Check sheet for the modelled part. Datum: model origin and axes. Units: mm. A direction names the side the tool comes from. Round coordinates to 2 decimals unless told otherwise and drop trailing zeros. Write each loop counter-clockwise with the first axis right and the second up, starting at its lowest first coordinate (ties: lowest second). Pieces come first, ordered by that corner, then holes. Notation, with made-up numbers: M -14.5,30.5 L 27.5,30.5 A6 ccw 27.5,39.5 Z; hole C 84.25,78.25 d11. An arc over 180 degrees is marked long. One line per item, written item: value.
from build123d import *

# Parameters (mm, degrees)
ESQUISSE1_W              = 80
ESQUISSE1_H              = 80
BOSS_EXTRU_1_DEPTH       = 20
ESQUISSE2_W              = 76
ESQUISSE2_H              = 76
BOSS_EXTRU_2_DEPTH       = 5
ESQUISSE3_W              = 72
ESQUISSE3_H              = 72
ENL_V_MAT_EXTRU_2_DEPTH  = 23
ESQUISSE4_W              = 15
ESQUISSE4_H              = 17.5
ESQUISSE4_W_2            = 17.5
ESQUISSE4_H_2            = 15
ENL_V_MAT_EXTRU_9_DEPTH  = 10
ESQUISSE7_R              = 2.5
ENL_V_MAT_EXTRU_4_DEPTH  = 10
ESQUISSE5_R              = 5
BOSS_EXTRU_6_DEPTH       = 10
ESQUISSE9_R              = 2
ENL_V_MAT_EXTRU_6_DEPTH  = 8
ESQUISSE10_W             = 2
ESQUISSE10_H             = 10
ENL_V_MAT_EXTRU_7_DEPTH  = 5
ESQUISSE11_OUTSIDE_W     = 105.174
ESQUISSE11_OUTSIDE_H     = 105.174
ESQUISSE11_OUTSIDE_W_2   = 75.6
ESQUISSE11_OUTSIDE_H_2   = 75.6
ENL_V_MAT_EXTRU_10_DEPTH = 3
BOSS_EXTRU_7_REACH       = 131.891
BOSS_EXTRU_7_START       = -15
ENL_V_MAT_EXTRU_11_DEPTH = 3


with BuildPart() as part:
    # Esquisse1 → Boss.-Extru.1 (new body)
    with BuildSketch(Plane(origin=(0, 0, 0), x_dir=(1, 0, 0), z_dir=(0, 1, 0))):
        with Locations((40, -40)):
            Rectangle(ESQUISSE1_W, ESQUISSE1_H)
    extrude(amount=BOSS_EXTRU_1_DEPTH)

    # Esquisse2 → Boss.-Extru.2 (add)
    with BuildSketch(Plane(origin=(0, 20, 0), x_dir=(1, 0, 0), z_dir=(0, 1, 0))):
        with Locations((40, -40)):
            Rectangle(ESQUISSE2_W, ESQUISSE2_H)
    extrude(amount=BOSS_EXTRU_2_DEPTH)

    # Esquisse3 → Enlèv. mat.-Extru.2 (cut)
    with BuildSketch(Plane(origin=(0, 25, 0), x_dir=(1, 0, 0), z_dir=(0, 1, 0))):
        with Locations((40, -40)):
            Rectangle(ESQUISSE3_W, ESQUISSE3_H)
    extrude(amount=-ENL_V_MAT_EXTRU_2_DEPTH, mode=Mode.SUBTRACT)

    # Esquisse4 → Enlèv. mat.-Extru.9 (cut)
    with BuildSketch(Plane.XZ):
        with Locations((40, 23.75)):
            Rectangle(ESQUISSE4_W, ESQUISSE4_H)
        with Locations((23.75, 40)):
            Rectangle(ESQUISSE4_W_2, ESQUISSE4_H_2)
        with Locations((40, 40)):
            Rectangle(ESQUISSE4_W, ESQUISSE4_H_2)
        with Locations((56.25, 40)):
            Rectangle(ESQUISSE4_W_2, ESQUISSE4_H_2)
        with Locations((40, 56.25)):
            Rectangle(ESQUISSE4_W, ESQUISSE4_H)
    extrude(amount=-ENL_V_MAT_EXTRU_9_DEPTH, mode=Mode.SUBTRACT)

    # Esquisse7 → Enlèv. mat.-Extru.4 (cut)
    with BuildSketch(Plane(origin=(0, 0, 0), x_dir=(-1, 0, 0), z_dir=(0, -1, 0))):
        with Locations(Location((-15, -15, 0), (0, 0, 90))):
            Circle(ESQUISSE7_R)
        with Locations(Location((-15, -65, 0), (0, 0, 90))):
            Circle(ESQUISSE7_R)
        with Locations(Location((-65, -15, 0), (0, 0, 90))):
            Circle(ESQUISSE7_R)
        with Locations(Location((-65, -65, 0), (0, 0, 90))):
            Circle(ESQUISSE7_R)
    extrude(amount=-ENL_V_MAT_EXTRU_4_DEPTH, mode=Mode.SUBTRACT)

    # Esquisse5 → Boss.-Extru.6 (add)
    with BuildSketch(Plane(origin=(0, 0, 0), x_dir=(-1, 0, 0), z_dir=(0, -1, 0))):
        with Locations(Location((-55, -25, 0), (0, 0, 90))):
            Circle(ESQUISSE5_R)
        with Locations(Location((-55, -55, 0), (0, 0, 90))):
            Circle(ESQUISSE5_R)
        with Locations(Location((-25, -55, 0), (0, 0, 90))):
            Circle(ESQUISSE5_R)
        with Locations(Location((-25, -25, 0), (0, 0, 90))):
            Circle(ESQUISSE5_R)
    extrude(amount=-BOSS_EXTRU_6_DEPTH)

    # Esquisse9 → Enlèv. mat.-Extru.6 (cut)
    with BuildSketch(Plane(origin=(0, 0, 0), x_dir=(-1, 0, 0), z_dir=(0, -1, 0))):
        with Locations(Location((-55, -25, 0), (0, 0, 90))):
            Circle(ESQUISSE9_R)
        with Locations(Location((-55, -55, 0), (0, 0, 90))):
            Circle(ESQUISSE9_R)
        with Locations(Location((-25, -25, 0), (0, 0, 90))):
            Circle(ESQUISSE9_R)
        with Locations(Location((-25, -55, 0), (0, 0, 90))):
            Circle(ESQUISSE9_R)
    extrude(amount=-ENL_V_MAT_EXTRU_6_DEPTH, mode=Mode.SUBTRACT)

    # Esquisse10 → Enlèv. mat.-Extru.7 (cut)
    with BuildSketch(Plane(origin=(0, 25, 0), x_dir=(1, 0, 0), z_dir=(0, 1, 0))):
        with Locations((3, -21)):
            Rectangle(ESQUISSE10_W, ESQUISSE10_H)
    extrude(amount=-ENL_V_MAT_EXTRU_7_DEPTH, mode=Mode.SUBTRACT)

    # Esquisse11 outside → Enlèv. mat.-Extru.10 (cut)
    with BuildSketch(Plane(origin=(0, 0, 0), x_dir=(-1, 0, 0), z_dir=(0, -1, 0))):
        with Locations((-40, -40)):
            Rectangle(ESQUISSE11_OUTSIDE_W, ESQUISSE11_OUTSIDE_H)
        with Locations((-40, -40)):
            Rectangle(ESQUISSE11_OUTSIDE_W_2, ESQUISSE11_OUTSIDE_H_2, mode=Mode.SUBTRACT)
    extrude(amount=-ENL_V_MAT_EXTRU_10_DEPTH, mode=Mode.SUBTRACT)

    # Esquisse14 → Boss.-Extru.7 (add, up to next)
    with BuildSketch(Plane(origin=(0, 20, 0), x_dir=(1, 0, 0), z_dir=(0, 1, 0)).offset(BOSS_EXTRU_7_START), mode=Mode.PRIVATE) as boss_extru_7_sk1:
        Polygon((76, -76), (76, -65.703145172), (66.703318607, -76), align=None)
    boss_extru_7_tool1 = extrude(boss_extru_7_sk1.sketch, amount=-BOSS_EXTRU_7_REACH, mode=Mode.PRIVATE) - part.part
    add(boss_extru_7_tool1.solids().sort_by_distance((72.901106, 5, 72.567715))[0])

    # Esquisse13 → Enlèv. mat.-Extru.11 (cut)
    with BuildSketch(Plane(origin=(0, 0, 0), x_dir=(-1, 0, 0), z_dir=(0, -1, 0))):
        Polygon((-63.5, -80), (-80, -63.5), (-80, -80), align=None)
    extrude(amount=-ENL_V_MAT_EXTRU_11_DEPTH, mode=Mode.SUBTRACT)


solid = part.part
Q1. Sectioned sample at B-B on y = 9. Enter the section's corners in (x, z), and give its area (3 significant figures).
Completed:
outline: M 0,0 L 80,0 L 80,80 L 0,80 Z; C 25,25 d10; C 25,55 d10; C 55,25 d10; C 55,55 d10; hole M 4,4 L 76,4 L 76,76 L 4,76 Z
area: 1,530 mm^2
Q2. Scan lines: line 1 (X direction, y = 3.25, z = 55); line 2 (X direction, y = 7.75, z = 35.5). Record each from-to range of solid material in increasing order. Write a range as [from, to].
Completed:
line 1: [0, 4], [20, 23], [27, 30], [50, 53], [57, 60], [76, 80]
line 2: [0, 4], [76, 80]
Q3. Depth check by flat-ended pin: P1, Ø11, axis at x = 55, z = 53, coming from the +Y side; P2, Ø2.5, axis at y = 2, z = 51.5, coming from the -X side; P3, Ø1.2, axis at x = 25.5, z = 55, coming from the -Y side; P4, Ø1.5, axis at x = 22.5, y = 23, coming from the +Z side. Enter the tip coordinate at first touch or a pass-through.
Completed:
P1: y = 10
P2: x = 0
P3: y = 8
P4: z = 78
Q4. Access from +Z, -Z, +X, -X, +Y, -Y to the whole of each face (thin tool, end or side, straight path). Record for faces 1 (the flat face through (25, 10, 55)), 2 (the flat face through (47.5, 1, 24)), 3 (the flat face through (25, 8, 25)).
Completed:
face 1: +Y
face 2: +Y, -Y
face 3: -Y
Q5. Sectioned sample at D-D on x = 51. Enter the section's corners in (y, z), and give its area (3 significant figures).
Completed:
outline: M 0,2.2 L 3,2.2 L 3,0 L 20,0 L 20,2 L 25,2 L 25,4 L 2,4 L 2,22 L 10,22 L 10,28 L 2,28 L 2,32.5 L 0,32.5 Z; M 0,47.5 L 2,47.5 L 2,52 L 10,52 L 10,58 L 2,58 L 2,76 L 25,76 L 25,78 L 20,78 L 20,80 L 3,80 L 3,77.8 L 0,77.8 Z
area: 377 mm^2
Q6. Sectioned sample at C-C on x = 34. Enter the section's corners in (y, z).
Completed:
outline: M 0,2.2 L 3,2.2 L 3,0 L 20,0 L 20,2 L 25,2 L 25,4 L 2,4 L 2,15 L 0,15 Z; M 0,65 L 2,65 L 2,76 L 25,76 L 25,78 L 20,78 L 20,80 L 3,80 L 3,77.8 L 0,77.8 Z
Q7. Draft check along X on faces 4 (the flat face through (36.9, 20, 78.3)), 5 (the flat face through (71.7, 1.5, 71.8)), 6 (the flat face through (31, 2, 31)). Enter one of: pulls with the +X half, pulls with the -X half, needs draft (parallel to the pull), parting line crosses it, or undercut.
Completed:
face 4: needs draft
face 5: pulls with the +X half
face 6: undercut
Q8. Sectioned sample at A-A on y = 4. State how many separate pieces and enclosed holes the cut face has, and give its area (3 significant figures).
Completed:
separate pieces: 5
enclosed holes: 5
area: 1,530 mm^2
